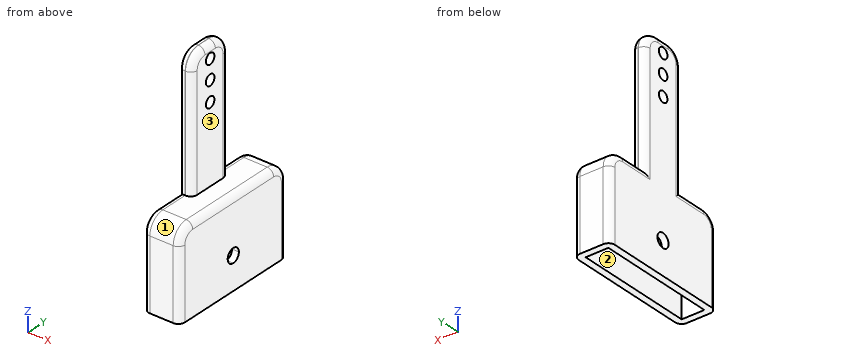
from build123d import *

# Parameters (mm, degrees)
F0_W          = 11.2
F0_H          = 41.2
F1_DEPTH      = 25
F3_DEPTH      = 2.1
F3_DEPTH_BACK = 9.1
F2_R          = 1.65
F4_DEPTH      = 2
F4_DEPTH_BACK = 2.1
F5_R          = 5
F6_R          = 2
F8_DEPTH      = 2.101
F8_DEPTH_BACK = 9.101


with BuildPart() as f1:
    # F0 (on Top) → F1 (new body)
    with BuildSketch(Plane.XY):
        with Locations((3.5, 18.5)):
            Rectangle(F0_W, F0_H)
        Polygon((7, 0), (0, 0), (0, 18.5), (0, 37), (7, 37), (7, 18.5), align=None, mode=Mode.SUBTRACT)
    extrude(amount=F1_DEPTH)

    # F2 (on Right) → F3 (join, two sides)
    with BuildSketch(Plane.YZ) as f3_sk:
        Polygon((-2.1, 26.8), (-2.1, 25), (39.1, 25), (39.1, 26.8), (25.5, 26.8), (18.5, 26.8), (11.5, 26.8), align=None)
    extrude(amount=-F3_DEPTH)
    extrude(f3_sk.sketch, amount=F3_DEPTH_BACK)

    # F2 (on Right) → F4 (join, two sides)
    with BuildSketch(Plane.YZ) as f4_sk:
        with BuildLine():
            Line((11.5, 61.8), (11.5, 26.8))
            Line((11.5, 26.8), (18.5, 26.8))
            Line((18.5, 26.8), (25.5, 26.8))
            Line((25.5, 26.8), (25.5, 61.8))
            ThreePointArc((25.5, 61.8), (24.0355339059, 65.3355339059), (20.5, 66.8))
            Line((20.5, 66.8), (16.5, 66.8))
            ThreePointArc((16.5, 66.8), (12.9644660941, 65.3355339059), (11.5, 61.8))
        make_face()
        with Locations((18.5, 50.5218207836)):
            Circle(F2_R, mode=Mode.SUBTRACT)
        with Locations((18.5, 56.8)):
            Circle(F2_R, mode=Mode.SUBTRACT)
        with Locations((18.5, 62.7918988466)):
            Circle(F2_R, mode=Mode.SUBTRACT)
    extrude(amount=F4_DEPTH)
    extrude(f4_sk.sketch, amount=-F4_DEPTH_BACK)

    # F5
    f5_edges = [f1.edges().sort_by_distance(p)[0] for p in [
        (3.5, -2.1, 26.8),
        (3.5, 39.1, 26.8),
    ]]
    fillet(f5_edges, radius=F5_R)

    # F6
    f6_edges = [f1.edges().sort_by_distance(p)[0] for p in [
        (-2.1, -2.1, 10.9),
        (-2.1, 39.1, 10.9),
        (9.1, -2.1, 10.9),
        (-2.1, 11.5, 44.3),
        (2, 11.5, 44.3),
    ]]
    fillet(f6_edges, radius=F6_R)

    # F7 (on Right) → F8 (cut, two sides)
    with BuildSketch(Plane.YZ) as f8_sk:
        with BuildLine():
            ThreePointArc((18.55, 7.85), (20.0702795796, 8.4797204204), (20.7, 10))
            ThreePointArc((20.7, 10), (17.0297204204, 11.5202795796), (18.55, 7.85))
        make_face()
    extrude(amount=-F8_DEPTH, mode=Mode.SUBTRACT)
    extrude(f8_sk.sketch, amount=F8_DEPTH_BACK, mode=Mode.SUBTRACT)


solid = f1.part
Can you work these out from the model? Positions are in its coordinate system, mm. Face numbers are marked on the shaded views. Give positions to 0.01 mm unless a question says otherwise; leave off trailing zeros. Write each loop counter-clockwise with the first axis right and the second up, starting at its lowest first coordinate (ties: lowest second). Pieces come first, ordered by that corner, then holes. Notation, with made-up numbers: (-40, 54) -> (-4, 54) arc R33 cw to (-4, 82) -> close; hole circle Ø9 at (16.25, 56). An arc over 180 degrees is marked (long way). Answer as a JSON object with one key per item and string values. Group by question number.
Item 1: Suppose I cut it at A-A (z = 56.8). Please give me the cut outline in (x, y), plus the area to 3 significant figures.
Item 2: I'm going to push flat-ended pins straight in: P1, Ø6, axis at x = 2, y = 25.5, coming from the +Z side; P2, Ø2, axis at y = 30, z = 28.5, coming from the -X side; P3, Ø1.5, axis at x = 3.5, y = 24, coming from the +Z side; P4, Ø2, axis at x = 3, y = 17, coming from the -Z side. Where does each tip first touch, or does it pass through?
Item 3: Suppose I cut it at D-D (x = 1). Please give me the cut outline in (y, z), plus the area to 3 significant figures.
Item 4: Please list where these lines run through material, in increasing order: line 1 (Z direction, x = -0.25, y = 18.5); line 2 (Z direction, x = 1, y = 18.5); line 3 (Z direction, x = 0.65, y = 18.5). Write a range as [from, to].
Item 5: We'd pull the mould along Y, two halves only. Please class the marked faces 1, 2 and 3: +Y half, -Y half, draft (parallel to the pull), parting line (faces both ways), or undercut.
Item 6: Suppose I cut it at B-B (y = 17.5). State how many separate pieces and enclosed holes the cut face has, plus the area to 3 significant figures.
Item 7: Suppose I cut it at C-C (x = 5.5). Please give me the cut outline in (y, z), plus the area to 3 significant figures.
Findings:
{
 "1": {"outline": "(-2.1, 13.5) arc R2 ccw to (-0.1, 11.5) -> (0, 11.5) arc R2 ccw to (2, 13.5) -> (2, 16.85) -> (-2.1, 16.85) -> close; (-2.1, 20.15) -> (2, 20.15) -> (2, 23.5) arc R2 ccw to (0, 25.5) -> (-0.1, 25.5) arc R2 ccw to (-2.1, 23.5) -> close", "area": "40.4 mm²"},
 "2": {"P1": "stops at z = 66.11", "P2": "passes through", "P3": "stops at z = 26.8", "P4": "stops at z = 25"},
 "3": {"outline": "(-2.1, 0) -> (0, 0) -> (0, 25) -> (37, 25) -> (37, 0) -> (39.1, 0) -> (39.1, 21.8) arc R5 ccw to (34.1, 26.8) -> (25.23, 26.8) -> (25.23, 61.8) arc R4.73 ccw to (20.5, 66.53) -> (16.5, 66.53) arc R4.73 ccw to (11.77, 61.8) -> (11.77, 26.8) -> (2.9, 26.8) arc R5 ccw to (-2.1, 21.8) -> close; hole circle Ø3.3 at (18.5, 50.52); hole circle Ø3.3 at (18.5, 56.8); hole circle Ø3.3 at (18.5, 62.79)", "area": "668 mm²"},
 "4": {"line 1": "z = [0, 7.85], [12.15, 48.87], [52.17, 55.15], [58.45, 61.14], [64.44, 66.79]", "line 2": "z = [25, 48.87], [52.17, 55.15], [58.45, 61.14], [64.44, 66.53]", "line 3": "z = [25, 48.87], [52.17, 55.15], [58.45, 61.14], [64.44, 66.69]"},
 "5": {"face 1": "-Y half", "face 2": "undercut", "face 3": "draft"},
 "6": {"separate pieces": "6", "enclosed holes": "0", "area": "239 mm²"},
 "7": {"outline": "(-2.1, 0) -> (0, 0) -> (0, 25) -> (37, 25) -> (37, 0) -> (39.1, 0) -> (39.1, 21.8) arc R5 ccw to (34.1, 26.8) -> (2.9, 26.8) arc R5 ccw to (-2.1, 21.8) -> close", "area": "168 mm²"}
}
